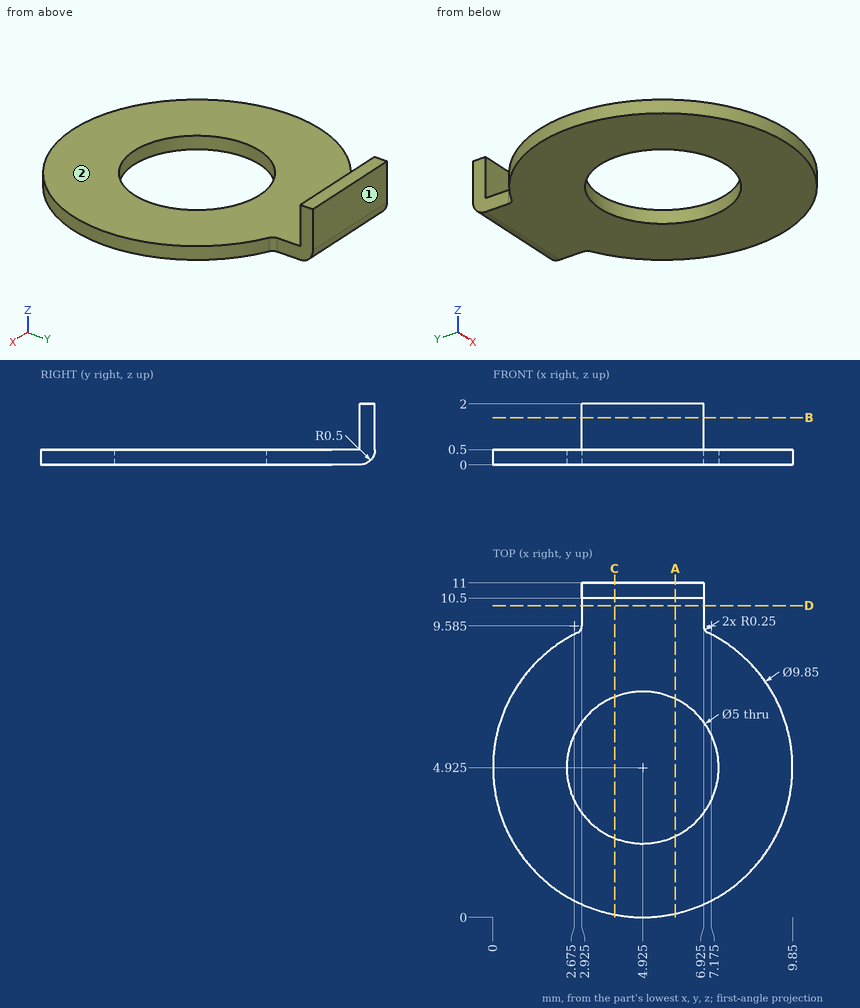
Could you check a few things on this drawing? It's one solid part, dimensions in mm from its lowest x, y, z. A direction names the side the tool comes from. Coordinates: 2 decimals unless noted, no trailing zeros. Loops run counter-clockwise (first coordinate to the right, second up) from the corner with the lowest first, then second, coordinate; pieces in that order, holes last. Notation, with made-up numbers: (22, -11.5) - (48, -11.5) arc R32 ccw to (48, 24.5) - close; hole circle Ø2 at (38.5, 27). An arc over 180 degrees is marked (long way). Return JSON: item names as keys, results as strings. Group by question number.
Item 1: If we section it at C-C on x = 4: Write out the boundary of the cut face in (y, z).
Item 2: If we section it at D-D on y = 10.25: Write out the boundary of the cut face in (x, z) (1 decimal).
Item 3: I need wall thicknesses on line 1 (Z direction, x = 8.75, y = 6); line 2 (Y direction, x = 4, z = 0.65); line 3 (Y direction, x = 4, z = 0.4). Which ranges of each line are inside material? Lowest first, please. Write a range as from..to.
Item 4: If we section it at B-B on z = 1.55: Write out the boundary of the cut face in (x, y) (1 decimal).
Item 5: On a 3-axis mill with a long thin cutter (end or side, diameter ignored), from which of +Z, -Z, +X, -X, +Y, -Y can I reach the whole of each face in a straight line? I mean the marked faces 1 and 2. Say none if no direction works.
Item 6: Will this pin go through, and if not, where does the flat tip stop? P1, Ø4, axis at x = 6.5, y = 6, coming from the +Z side.
Item 7: If we section it at A-A on x = 6: Write out the boundary of the cut face in (y, z).
Calculated:
{
 "1": {"outline": "(0.09, 0) - (2.6, 0) - (2.6, 0.5) - (0.09, 0.5) - close; (7.25, 0) - (10.5, 0) arc R0.5 ccw to (11, 0.5) - (11, 2) - (10.5, 2) - (10.5, 0.5) - (7.25, 0.5) - close"},
 "2": {"outline": "(2.9, 0) - (6.9, 0) - (6.9, 0.5) - (2.9, 0.5) - close"},
 "3": {"line 1": "z = 0..0.5", "line 2": "y = 10.5..11", "line 3": "y = 0.09..2.6, 7.25..10.99"},
 "4": {"outline": "(2.9, 10.5) - (6.9, 10.5) - (6.9, 11) - (2.9, 11) - close"},
 "5": {"face 1": "+Z, -Z, +X, -X, +Y", "face 2": "+Z, +X, -X, -Y"},
 "6": {"P1": "stops at z = 0.5"},
 "7": {"outline": "(0.12, 0) - (2.67, 0) - (2.67, 0.5) - (0.12, 0.5) - close; (7.18, 0) - (10.5, 0) arc R0.5 ccw to (11, 0.5) - (11, 2) - (10.5, 2) - (10.5, 0.5) - (7.18, 0.5) - close"}
}
